from build123d import *

# Parameters (mm, degrees)
PAD002_DEPTH    = 847
SKETCH006_R     = 4.5
POCKET003_DEPTH = 5
SKETCH008_W     = 36
SKETCH008_H     = 847
POCKET005_DEPTH = 5


with BuildPart() as part:
    # Sketch005 → Pad002 (new body)
    with BuildSketch(Plane.XY):
        with BuildLine():
            Line((-19.5, 11), (19.5, 11))
            ThreePointArc((22, 8.5), (21.267767, 10.267767), (19.5, 11))
            Line((22, 8.5), (22, -8.5))
            ThreePointArc((19.5, -11), (21.267767, -10.267767), (22, -8.5))
            Line((19.5, -11), (-19.5, -11))
            ThreePointArc((-22, -8.5), (-21.267767, -10.267767), (-19.5, -11))
            Line((-22, -8.5), (-22, 8.5))
            ThreePointArc((-19.5, 11), (-21.267767, 10.267767), (-22, 8.5))
        make_face()
        with BuildLine():
            Line((-19.5, 10), (19.5, 10))
            ThreePointArc((21, 8.5), (20.56066, 9.56066), (19.5, 10))
            Line((21, 8.5), (21, -8.5))
            ThreePointArc((19.5, -10), (20.56066, -9.56066), (21, -8.5))
            Line((19.5, -10), (-19.5, -10))
            ThreePointArc((-21, -8.5), (-20.56066, -9.56066), (-19.5, -10))
            Line((-21, -8.5), (-21, 8.5))
            ThreePointArc((-19.5, 10), (-20.56066, 9.56066), (-21, 8.5))
        make_face(mode=Mode.SUBTRACT)
    extrude(amount=PAD002_DEPTH)

    # Sketch006 (on Face7 of Pad002) → Pocket003 (cut)
    with BuildSketch(Plane.XZ.offset(11)):
        with Locations((0, 9)):
            Circle(SKETCH006_R)
        with Locations((0, 838)):
            Circle(SKETCH006_R)
    extrude(amount=-POCKET003_DEPTH, mode=Mode.SUBTRACT)

    # Sketch008 (on Face7 of Pocket003) → Pocket005 (cut)
    with BuildSketch(Plane(origin=(0, 11, 0), x_dir=(-1, 0, 0), z_dir=(0, 1, 0))):
        with Locations((0, 423.5)):
            Rectangle(SKETCH008_W, SKETCH008_H)
    extrude(amount=-POCKET005_DEPTH, mode=Mode.SUBTRACT)


solid = part.part
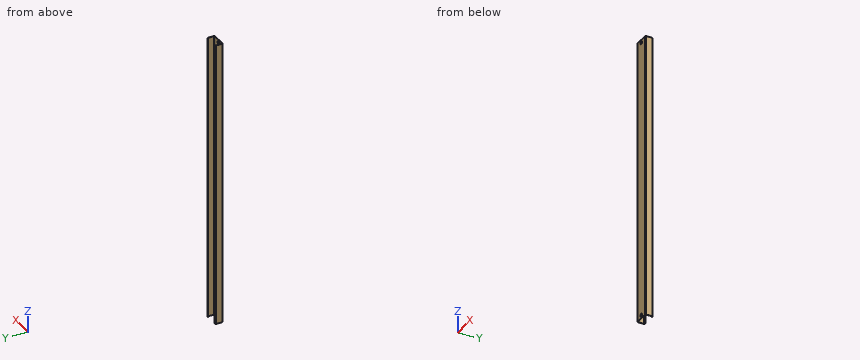
Read the model definition and answer for the solid it produces. Units are mm, in the model's axes. Round coordinates to 2 decimals unless told otherwise and drop trailing zeros. Loops run counter-clockwise (first coordinate to the right, second up) from the corner with the lowest first, then second, coordinate; pieces in that order, holes last.
Q1. Section A-A on y = 2.5 is taken. Write down the section's boundary in (x, z).
Q2. Section B-B on z = 99 is taken. Write down the section's boundary in (x, y).
Q3. Each of these flat-tipped pins is pushed along its axis until it touches: pin 1 (1 mm diameter, centred on x = -6, z = 455.5, fed in from +Y); pin 2 (1.1 mm diameter, centred on y = 10.5, z = 544, fed in from -X); pin 3 (8 mm diameter, centred on x = 0, z = 838, fed in from +Y); pin 4 (11.5 mm diameter, centred on x = 0, z = 9, fed in from -Y). Where does it stop, or does it pass through?
Q4. Consider probe 1 along Z at (x, y) = (0, -10.25); probe 2 along X at (y, z) = (-1.5, 307); probe 3 along X at (y, z) = (-10.4, 838). Determine where each line is inside the solid, lowest interval first.
Output:
1. outline: (-22, 0) - (-21, 0) - (-21, 847) - (-22, 847) - close; (21, 0) - (22, 0) - (22, 847) - (21, 847) - close
2. outline: (-22, -8.5) arc R2.5 ccw to (-19.5, -11) - (19.5, -11) arc R2.5 ccw to (22, -8.5) - (22, 8.5) arc R2.5 ccw to (19.5, 11) - (18, 11) - (18, 10) - (19.5, 10) arc R1.5 cw to (21, 8.5) - (21, -8.5) arc R1.5 cw to (19.5, -10) - (-19.5, -10) arc R1.5 cw to (-21, -8.5) - (-21, 8.5) arc R1.5 cw to (-19.5, 10) - (-18, 10) - (-18, 11) - (-19.5, 11) arc R2.5 ccw to (-22, 8.5) - close
3. pin 1: stops at y = -10
3. pin 2: stops at x = -21.54
3. pin 3: passes through
3. pin 4: stops at y = -11
4. probe 1: z = 0 to 4.5, 13.5 to 833.5, 842.5 to 847
4. probe 2: x = -22 to -21, 21 to 22
4. probe 3: x = -21.12 to -4.5, 4.5 to 21.12
